```python
from build123d import *

# Parameters (mm, degrees)
CUT_EXTRUDE1_DEPTH      = 17.015617378
CUT_EXTRUDE1_DEPTH_BACK = 17.015617378
SKETCH2_R               = 4
CHAMFER1_SIZE           = 0.2
CUT_EXTRUDE2_DEPTH      = 5
CUT_EXTRUDE2_DEPTH_BACK = 5
SKETCH4_R               = 1.5


with BuildPart() as part:
    # Sketch1 → Revolve1 (revolve)
    with BuildSketch(Plane.XY, mode=Mode.PRIVATE) as revolve1_sk:
        Polygon((0, 5.5), (-5, 5.5), (-5, 7.5), (-6, 7.5), (-6, 0), (0, 0), align=None)
    revolve1 = revolve(revolve1_sk.sketch.rotate(Axis((-6, 0, 0), (1, 0, 0)), 90), axis=Axis((-6, 0, 0), (1, 0, 0)))

    # Mirror1: Revolve1 across plane
    add(revolve1.mirror(Plane(origin=(0, 0, 0), x_dir=(0, 0, 1), z_dir=(1, 0, 0))))

    # Sketch2 → Cut-Extrude1 (cut, two sides: drawn at the far end of the back side and taken through both)
    with BuildSketch(Plane.ZY.offset(6).offset(-CUT_EXTRUDE1_DEPTH_BACK)):
        Circle(SKETCH2_R)
    extrude(amount=CUT_EXTRUDE1_DEPTH + CUT_EXTRUDE1_DEPTH_BACK, mode=Mode.SUBTRACT)

    # Chamfer1
    chamfer1_edges = [part.edges().sort_by_distance(p)[0] for p in [
        (6, 0, -7.5),
        (6, 0, -4),
        (-6, 0, -4),
        (-6, 0, -7.5),
    ]]
    chamfer(chamfer1_edges, length=CHAMFER1_SIZE)

    # Sketch4 → Cut-Extrude2 (cut, two sides: drawn at the far end of the back side and taken through both)
    with BuildSketch(Plane(origin=(0, -3.464101615, 2), x_dir=(-1, 0, 0), z_dir=(0, 0.866025403784438, -0.500000000000001)).offset(-CUT_EXTRUDE2_DEPTH_BACK)):
        with Locations(Location((0, 0, 0), (0, 0, 90))):
            Circle(SKETCH4_R)
    extrude(amount=CUT_EXTRUDE2_DEPTH + CUT_EXTRUDE2_DEPTH_BACK, mode=Mode.SUBTRACT)


solid = part.part
```
The listing builds one solid part. Answer for the finished solid, in the listing's coordinates (mm). A direction names the side the tool comes from. Give positions to 0.01 mm unless a question says otherwise; leave off trailing zeros. Write each loop counter-clockwise with the first axis right and the second up, starting at its lowest first coordinate (ties: lowest second). Pieces come first, ordered by that corner, then holes. Notation, with made-up numbers: (9.5, -31.75) -> (29.5, -31.75) arc R32 ccw to (29.5, 7.25) -> close; hole circle Ø11 at (47.5, 37). An arc over 180 degrees is marked (long way). Write item = value, one per line. Start each with the question number.
1) Each of these flat-tipped pins is pushed along its axis until it touches: pin 1 (1 mm diameter, centred on x = -2, y = -0.5, fed in from +Z); pin 2 (4.5 mm diameter, centred on y = -0.5, z = 3, fed in from -X); pin 3 (1.5 mm diameter, centred on x = 1.5, z = 0.5, fed in from -Y); pin 4 (1.5 mm diameter, centred on x = -0.5, y = -4.5, fed in from +Z). Where does it stop, or does it pass through?
2) The part is cut by section D-D, the plane x = 1. Determine the outline of the cut face in (y, z), and give its area (3 significant figures).
3) The part is cut by section A-A, the plane z = 0. Determine the outline of the cut face in (x, y).
4) The part is cut by section C-C, the plane x = -3.5. Determine the outline of the cut face in (y, z).
5) Straight lines are drawn through the part: line 1 along Y through (x, z) = (1, 0); line 2 along X through (y, z) = (5.25, -2.75); line 3 along Z through (x, y) = (-3.75, -1). For each, find the intervals that lie inside material, in ascending order.
6) Which of the six approach directions +Z, -Z, +X, -X, +Y, -Y give full straight-line access (tool end or side, diameter ignored) to faces 1 (the face through (5.406, -6.324, 4.032)), 2 (the face through (5, -4, 4))?
7) Determine the mould class of faces 3 (the face through (-6, 3.1, 3.1)), 4 (the face through (-1.33, -3.65, 2.91)), 5 (the face through (-5.406, -6.324, 4.032)), 6 (the face through (-5, -4, 4)) for opening direction X: +X half, -X half, draft (parallel to the pull), parting line (faces both ways), or undercut.
Solutions:
q1.pin_1 = 5.5
q1.pin_2 = -6
q1.pin_3 = -5.5
q1.pin_4 = 4.02
q2.outline = (-5.22, 1.72) arc R5.5 ccw (long way) to (-4.1, 3.66) -> (-2.77, 2.89) arc R4 cw (long way) to (-3.89, 0.95) -> close
q2.area = 41.4 mm²
q3.outline = (-6, -7.3) -> (-5.8, -7.5) -> (-5, -7.5) -> (-5, -5.5) -> (5, -5.5) -> (5, -7.5) -> (5.8, -7.5) -> (6, -7.3) -> (6, -4.2) -> (5.8, -4) -> (-5.8, -4) -> (-6, -4.2) -> close; (-6, 4.2) -> (-5.8, 4) -> (5.8, 4) -> (6, 4.2) -> (6, 7.3) -> (5.8, 7.5) -> (5, 7.5) -> (5, 5.5) -> (-5, 5.5) -> (-5, 7.5) -> (-5.8, 7.5) -> (-6, 7.3) -> close
q4.outline = circle Ø11 at (0, 0); hole circle Ø8 at (0, 0)
q5.line_1 = -5.5 to -4, 4 to 5.5
q5.line_2 = -6 to -5, 5 to 6
q5.line_3 = -5.41 to -3.87, 3.87 to 5.41
q6.face_1 = +X, -X
q6.face_2 = none
q7.face_3 = -X half
q7.face_4 = undercut
q7.face_5 = draft
q7.face_6 = undercut
